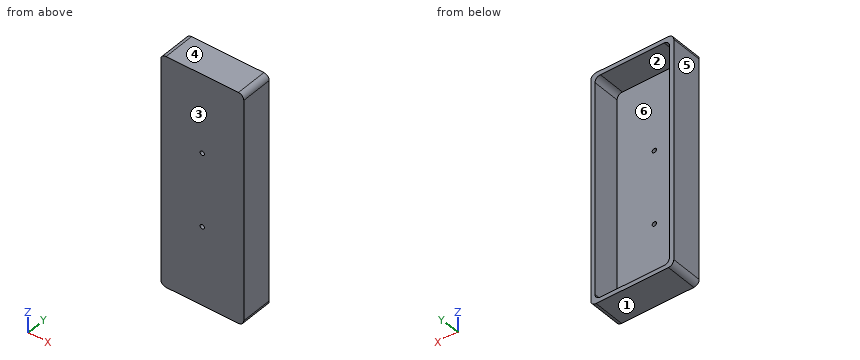
Autodesk Inventor part; units mm, degrees
ref_plane "YZ Plane" through (0, 0, 0) normal (1, 0, 0) x (0, 1, 0)
ref_plane "XZ Plane" through (0, 0, 0) normal (0, 1, 0) x (-1, 0, 0)
ref_plane "XY Plane" through (0, 0, 0) normal (0, 0, 1) x (1, 0, 0)
sketch "Sketch1" plane through (0, 0, 0) normal (0, 1, 0) x (-1, 0, 0)
  line L0 (5, 0) -> (73, 0)
  line L1 (78, -5) -> (78, -212)
  line L2 (73, -217) -> (5, -217)
  line L3 (0, -212) -> (0, -5)
  line L4 (69, -4) -> (9, -4)
  line L5 (4, -9) -> (4, -208)
  line L6 (9, -213) -> (69, -213)
  line L7 (74, -208) -> (74, -9)
  line L8 (74, -4) -> (4, -213) construction
  line L9 (4, -4) -> (74, -213) construction
  arc A0 (78, -5) -> (73, 0) centre (73, -5) ccw
  arc A1 (5, 0) -> (0, -5) centre (5, -5) ccw
  arc A2 (73, -217) -> (78, -212) centre (73, -212) ccw
  arc A3 (0, -212) -> (5, -217) centre (5, -212) ccw
  arc A4 (74, -9) -> (69, -4) centre (69, -9) ccw
  arc A5 (9, -4) -> (4, -9) centre (9, -9) ccw
  arc A6 (69, -213) -> (74, -208) centre (69, -208) ccw
  arc A7 (4, -208) -> (9, -213) centre (9, -208) ccw
  circle A8 centre (39, -143) radius 2
  line L10 (39, -108.5) -> (37, -108.5)
  circle A9 centre (39, -74) radius 2
  point P0 (0, 0)
  point P1 (78, -217)
  point P2 (78, 0)
  point P3 (0, -217)
  dimension "d0" = 78
  dimension "d1" = 217
  dimension "d2" = 70
  dimension "d3" = 209
  dimension "d4" = 5
  dimension "d5" = 5
  dimension "d10" = 4
  dimension "d14" = 69
extrude "Extrusion1" add sketch "Sketch1" along normal blind 30 contours L0 A0 L1 A2 L2 A3 L3 A1
extrude "Extrusion2" add sketch "Sketch1" along normal blind 4 contours A4 L7 A6 L6 A7 L5 A5 L4 | A8 | A9
extrude "Extrusion3" cut sketch "Sketch1" along normal blind 4 contours A8 | A9
properties part number "Kepala"
Work out the finished part from the listing and answer in its coordinate system (mm). Face numbers are marked on the shaded views. A direction names the side the tool comes from. Coordinates: 2 decimals unless noted, no trailing zeros. Loops run counter-clockwise (first coordinate to the right, second up) from the corner with the lowest first, then second, coordinate; pieces in that order, holes last.
1) For a pull along Z with two mould halves and no side action, classify the marked faces 1, 2, 3 and 4 as +Z half, -Z half, draft (parallel to the pull), parting line (faces both ways), or undercut.
Results:
face 1: -Z half
face 2: undercut
face 3: draft
face 4: +Z half
2) Flat-ended cylindrical pins translate along their axes: pin 1 (8 mm diameter, centred on y = 22.5, z = -96.5, fed in from +X); pin 2 (2 mm diameter, centred on x = -62, z = -181, fed in from +Y). Find the tip coordinate at first contact, or state that the pin passes through.
Results:
pin 1: stops at x = 0
pin 2: stops at y = 4
3) Section C-C (y = 14.5) is taken. Give the vertices of the cut face in (x, z), plus the area to 3 significant figures.
Results:
outline: (-78, -212) arc R5 ccw to (-73, -217) - (-5, -217) arc R5 ccw to (0, -212) - (0, -5) arc R5 ccw to (-5, 0) - (-73, 0) arc R5 ccw to (-78, -5) - close; hole (-74, -208) arc R5 ccw to (-69, -213) - (-9, -213) arc R5 ccw to (-4, -208) - (-4, -9) arc R5 ccw to (-9, -4) - (-69, -4) arc R5 ccw to (-74, -9) - close
area: 2,300 mm2
4) Section D-D (z = -100) is taken. Give the vertices of the cut face in (x, y), plus the area to 3 significant figures.
Results:
outline: (-78, 0) - (0, 0) - (0, 30) - (-4, 30) - (-4, 4) - (-74, 4) - (-74, 30) - (-78, 30) - close
area: 520 mm2
5) Section A-A (x = -39) is taken. Give the vertices of the cut face in (y, z), plus the area to 3 significant figures.
Results:
outline: (0, -217) - (30, -217) - (30, -213) - (4, -213) - (4, -145) - (0, -145) - close; (0, -141) - (4, -141) - (4, -76) - (0, -76) - close; (0, -72) - (4, -72) - (4, -4) - (30, -4) - (30, 0) - (0, 0) - close
area: 1,040 mm2
6) Consider probe 1 along Z at (x, y) = (-39, 2.05); probe 2 along Z at (x, y) = (-61.5, 15); probe 3 along X at (y, z) = (1.3, -143). Determine where each line is inside the solid, lowest interval first.
Results:
probe 1: z = -217 to -145, -141 to -76, -72 to 0
probe 2: z = -217 to -213, -4 to 0
probe 3: x = -78 to -41, -37 to 0
7) For the marked faces 5 and 6, determine the directions among +Z, -Z, +X, -X, +Y, -Y from which every point of the face is accessible in a straight line to the end or side of a thin tool.
Results:
face 5: +Z, -Z, -X, +Y, -Y
face 6: +Y
8) Section B-B (z = -143) is taken. Give the vertices of the cut face in (x, y), plus the area to 3 significant figures.
Results:
outline: (-78, 0) - (-41, 0) - (-41, 4) - (-74, 4) - (-74, 30) - (-78, 30) - close; (-37, 0) - (0, 0) - (0, 30) - (-4, 30) - (-4, 4) - (-37, 4) - close
area: 504 mm2
